Geometry: see drawing. Coordinates: mm, zero at the bounding-box minimum. Coordinates: 2 decimals unless noted, no trailing zeros. Loops run counter-clockwise (first coordinate to the right, second up) from the corner with the lowest first, then second, coordinate; pieces in that order, holes last. Notation, with made-up numbers: (-35.75, 20.5) -> (19.25, 20.5) arc R15 cw to (19.25, 39.5) -> close; hole circle Ø10 at (20.5, 48.25). An arc over 180 degrees is marked (long way). Answer as a JSON object with one key per item and string values.
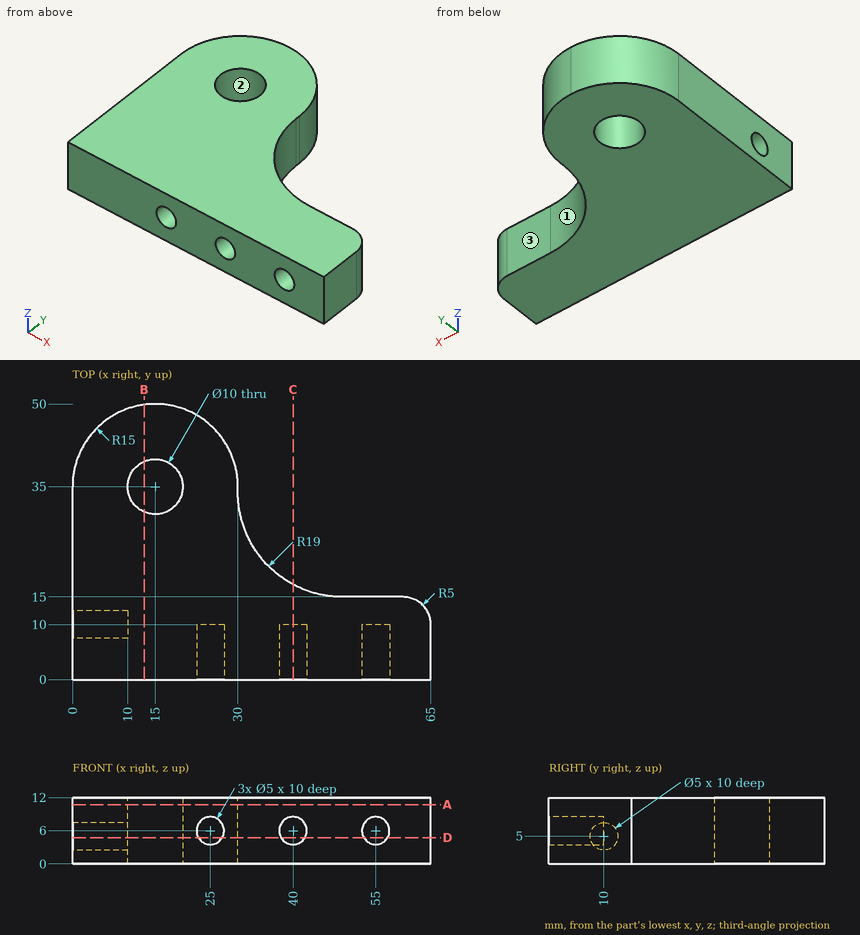
1. Section query C-C (x = 40). Return loops of the section in (y, z).
Reply:
{"outline": "(0, 0) -> (17.27, 0) -> (17.27, 12) -> (0, 12) -> (0, 8.5) -> (10, 8.5) -> (10, 3.5) -> (0, 3.5) -> close"}
2. Line query: line 1 along X through (y, z) = (8, 6); line 2 along X through (y, z) = (4.5, 6); line 3 along Y through (x, z) = (55, 5). Output: solid intervals per line, ascending.
Reply:
{"line 1": "x = 10 to 22.5, 27.5 to 37.5, 42.5 to 52.5, 57.5 to 65", "line 2": "x = 0 to 22.5, 27.5 to 37.5, 42.5 to 52.5, 57.5 to 65", "line 3": "y = 10 to 15"}
3. Section query A-A (z = 10.75). Return loops of the section in (x, y), plus the area to 3 significant figures.
Reply:
{"outline": "(0, 0) -> (65, 0) -> (65, 10) arc R5 ccw to (60, 15) -> (49, 15) arc R19 cw to (30, 34) -> (30, 35) arc R15 ccw to (0, 35) -> close; hole circle Ø10 at (15, 35)", "area": "1,920 mm2"}
4. Section query B-B (x = 13). Return loops of the section in (y, z), plus the area to 3 significant figures.
Reply:
{"outline": "(0, 0) -> (30.42, 0) -> (30.42, 12) -> (0, 12) -> close; (39.58, 0) -> (49.87, 0) -> (49.87, 12) -> (39.58, 12) -> close", "area": "488 mm2"}
5. Section query D-D (z = 4.75). Return loops of the section in (x, y), plus the area to 3 significant figures.
Reply:
{"outline": "(0, 0) -> (22.83, 0) -> (22.83, 10) -> (27.17, 10) -> (27.17, 0) -> (37.83, 0) -> (37.83, 10) -> (42.17, 10) -> (42.17, 0) -> (52.83, 0) -> (52.83, 10) -> (57.17, 10) -> (57.17, 0) -> (65, 0) -> (65, 10) arc R5 ccw to (60, 15) -> (49, 15) arc R19 cw to (30, 34) -> (30, 35) arc R15 ccw to (0, 35) -> (0, 12.49) -> (10, 12.49) -> (10, 7.51) -> (0, 7.51) -> close; hole circle Ø10 at (15, 35)", "area": "1,740 mm2"}
6. Mould query, pull axis X, two halves, no side actions, for the marked faces 1, 2 and 3. Classes: pulls with the +X half, pulls with the -X half, needs draft (parallel to the pull), parting line crosses it, or undercut.
Reply:
{"face 1": "pulls with the +X half", "face 2": "undercut", "face 3": "needs draft"}
7. Pin query (flat end, axial travel): P1, Ø3, axis at x = 40, z = 6, coming from the -Y side; P2, Ø3, axis at y = 22.5, z = 7.5, coming from the +X side; P3, Ø6, axis at x = 25, z = 6, coming from the +Y side; P4, Ø9, axis at x = 15, y = 35, coming from the +Z side. Return the tip coordinate at first contact, or that it passes through.
Reply:
{"P1": "stops at y = 10", "P2": "stops at x = 35.14", "P3": "stops at y = 48.27", "P4": "passes through"}
